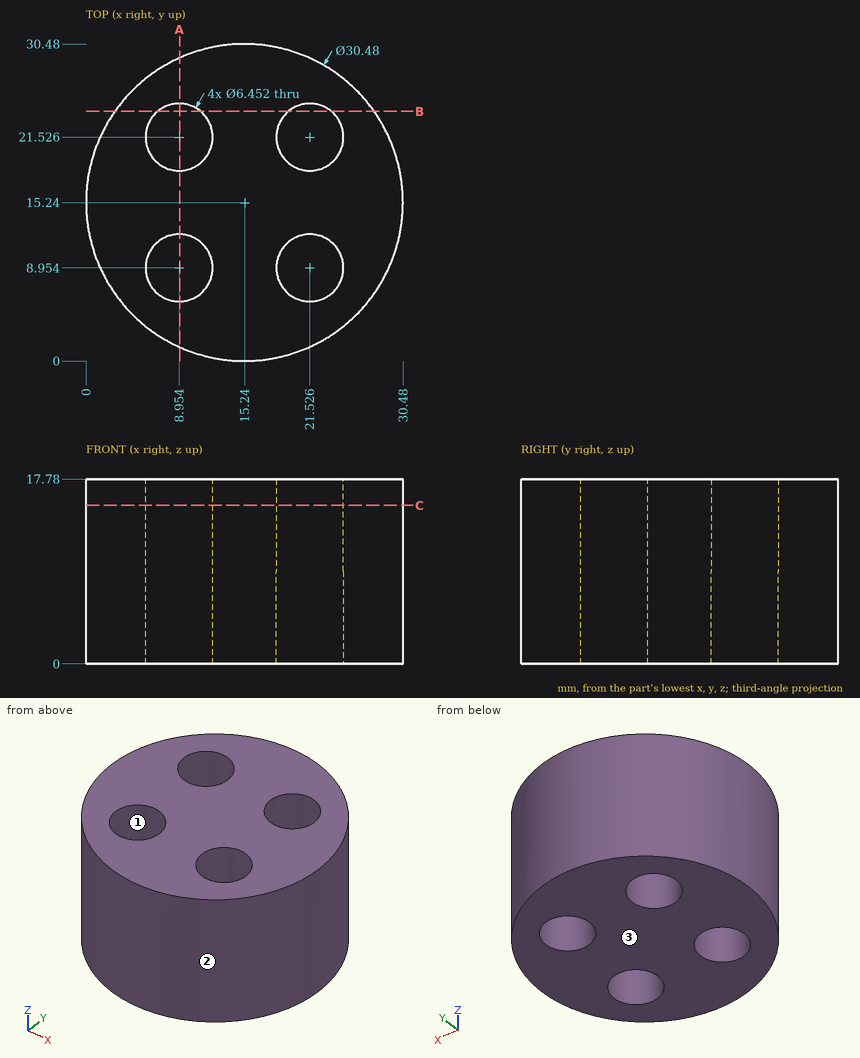
Input: dimensioned drawing with shaded views. Units: mm. Origin: part minimum x, y, z. Round coordinates to 2 decimals unless told otherwise and drop trailing zeros. Order: outer loops, then holes, each group sorted by start corner. A loop starts at its lowest first (then second) coordinate and runs counter-clockwise, first axis right, second up.
1. Cut plane C-C, the plane z = 15.25. Output: boundary loops of the cut face in (x, y) (1 decimal).
The answers:
outline: circle Ø30.5 at (15.2, 15.2); hole circle Ø6.5 at (9, 9); hole circle Ø6.5 at (9, 21.5); hole circle Ø6.5 at (21.5, 9); hole circle Ø6.5 at (21.5, 21.5)
2. Cut plane A-A, the plane x = 9. Output: boundary loops of the cut face in (y, z).
The answers:
outline: (1.34, 0) - (5.73, 0) - (5.73, 17.78) - (1.34, 17.78) - close; (12.18, 0) - (18.3, 0) - (18.3, 17.78) - (12.18, 17.78) - close; (24.75, 0) - (29.14, 0) - (29.14, 17.78) - (24.75, 17.78) - close
3. Cut plane B-B, the plane y = 24. Output: boundary loops of the cut face in (x, z).
The answers:
outline: (2.77, 0) - (6.88, 0) - (6.88, 17.78) - (2.77, 17.78) - close; (11.02, 0) - (19.46, 0) - (19.46, 17.78) - (11.02, 17.78) - close; (23.6, 0) - (27.71, 0) - (27.71, 17.78) - (23.6, 17.78) - close
4. Material intervals for line 1 (X direction, y = 23, z = 15.5) (1 decimal); line 2 (X direction, y = 19.5, z = 3) (1 decimal); line 3 (Y direction, x = 9, z = 9) (1 decimal), sorted ascending.
The answers:
line 1: x = 2.1 to 6.1, 11.8 to 18.7, 24.4 to 28.4
line 2: x = 0.6 to 6.4, 11.5 to 19, 24 to 29.9
line 3: y = 1.3 to 5.7, 12.2 to 18.3, 24.8 to 29.1
5. Pin query (flat end, axial travel): P1, Ø1.5, axis at y = 17.5, z = 15.5, coming from the +X side (1 decimal); P2, Ø1, axis at y = 10, z = 6.5, coming from the -X side; P3, Ø1, axis at x = 12, z = 12.5, coming from the -Y side. Return the tip coordinate at first contact, or that it passes through.
The answers:
P1: stops at x = 30.4
P2: stops at x = 0.76
P3: stops at y = 0.25
6. Mould query, pull axis X, two halves, no side actions, for the marked faces 1, 2 and 3. Classes: released by +X, released by -X, zero draft, split by the parting line, or undercut.
The answers:
face 1: undercut
face 2: split by the parting line
face 3: zero draft
